The model under review builds one solid part; all positions refer to its coordinate system, in mm. A direction names the side the tool comes from. Coordinates: 2 decimals unless noted, no trailing zeros. Order: outer loops, then holes, each group sorted by start corner. A loop starts at its lowest first (then second) coordinate and runs counter-clockwise, first axis right, second up. Notation, with made-up numbers: M -40,41 L -4,41 A11 cw -4,53 Z; hole C 38.25,70.25 d1. An arc over 180 degrees is marked long. Write each question's results on one line, items separated by ' | '.
from build123d import *

# Parameters (mm, degrees)
SALIENTE_EXTRUIR1_DEPTH = 6.8
CROQUIS2_W              = 9
CROQUIS2_H              = 2.8
CORTAR_EXTRUIR1_DEPTH   = 18.969669092
REDONDEO1_R             = 0.5
REDONDEO2_R             = 0.5
REDONDEO3_R             = 0.5
REDONDEO4_R             = 0.5


with BuildPart() as part:
    # Croquis1 → Saliente-Extruir1 (new body)
    with BuildSketch(Plane(origin=(0, 0, 0), x_dir=(1, 0, 0), z_dir=(0, 1, 0))):
        with BuildLine():
            Line((0, 0), (0, 14))
            Line((0, 14), (1, 14))
            Line((1, 14), (1, 1.5))
            Line((1, 1.5), (3.5, 1.5))
            Line((3.5, 1.5), (3.5, 9.4))
            Line((3.5, 9.4), (1.5, 9.4))
            Line((1.5, 9.4), (1.5, 11.6))
            Line((1.5, 11.6), (3.5, 11.6))
            Line((3.5, 11.6), (3.5, 17.969669092))
            Line((3.5, 17.969669092), (4.5, 17.969669092))
            Line((4.5, 17.969669092), (4.5, 2.5))
            ThreePointArc((4.5, 2.5), (4.792893219, 1.792893219), (5.5, 1.5))
            Line((5.5, 1.5), (12.5, 1.5))
            ThreePointArc((12.5, 1.5), (13.207106781, 1.792893219), (13.5, 2.5))
            Line((13.5, 2.5), (13.5, 17.969669092))
            Line((13.5, 17.969669092), (14.5, 17.969669092))
            Line((14.5, 17.969669092), (14.5, 11.6))
            Line((14.5, 11.6), (16.5, 11.6))
            Line((16.5, 11.6), (16.5, 9.4))
            Line((16.5, 9.4), (14.5, 9.4))
            Line((14.5, 9.4), (14.5, 1.5))
            Line((14.5, 1.5), (17, 1.5))
            Line((17, 1.5), (17, 14))
            Line((17, 14), (18, 14))
            Line((18, 14), (18, 0))
            Line((18, 0), (0, 0))
        make_face()
    extrude(amount=SALIENTE_EXTRUIR1_DEPTH)

    # Croquis2 → Cortar-Extruir1 (cut, through all)
    with BuildSketch(Plane.XY):
        with Locations((9, 3.4)):
            Rectangle(CROQUIS2_W, CROQUIS2_H)
    extrude(amount=-CORTAR_EXTRUIR1_DEPTH, mode=Mode.SUBTRACT)

    # Redondeo1
    redondeo1_edges = [part.edges().sort_by_distance(p)[0] for p in [
        (16.5, 3.4, -11.6),
    ]]
    fillet(redondeo1_edges, radius=REDONDEO1_R)

    # Redondeo2
    redondeo2_edges = [part.edges().sort_by_distance(p)[0] for p in [
        (16.5, 3.4, -9.4),
    ]]
    fillet(redondeo2_edges, radius=REDONDEO2_R)

    # Redondeo3
    redondeo3_edges = [part.edges().sort_by_distance(p)[0] for p in [
        (1.5, 3.4, -9.4),
    ]]
    fillet(redondeo3_edges, radius=REDONDEO3_R)

    # Redondeo4
    redondeo4_edges = [part.edges().sort_by_distance(p)[0] for p in [
        (1.5, 3.4, -11.6),
    ]]
    fillet(redondeo4_edges, radius=REDONDEO4_R)


solid = part.part
1) Take a section at A-A on x = 9. State the section outline as (y, z) points.
Solutions:
outline: M 0,-1.5 L 2,-1.5 L 2,0 L 0,0 Z; M 4.8,-1.5 L 6.8,-1.5 L 6.8,0 L 4.8,0 Z
2) Take a section at C-C on z = -9. State the section outline as (x, y) points.
Solutions:
outline: M 0,0 L 1,0 L 1,6.8 L 0,6.8 Z; M 3.5,0 L 4.5,0 L 4.5,6.8 L 3.5,6.8 Z; M 13.5,0 L 14.5,0 L 14.5,6.8 L 13.5,6.8 Z; M 17,0 L 18,0 L 18,6.8 L 17,6.8 Z
3) For faces 4 (the flat face through (14, 3, -17.97)), 5 (the flat face through (14.5, 3, -15)), 6 (the flat face through (9, 5, 0)), 7 (the flat face through (3, 3, -9.4)), 8 (the flat face through (17.5, 3.4, -14)), list the 3-axis set-ups (+Z, -Z, +X, -X, +Y, -Y) from which the entire face can be reached by the end or side of a thin tool; tool diameter is ignored.
Solutions:
face 4: -Z, +X, -X, +Y, -Y | face 5: -Z, +Y, -Y | face 6: +Z, +X, -X, +Y, -Y | face 7: +Y, -Y | face 8: -Z, +X, +Y, -Y
4) To check wall thickness, follow line 1 along X through (y, z) = (4, -8); line 2 along Z through (x, y) = (2, 4.75); line 3 along X through (y, z) = (1.5, -10.75). State the ranges of each line that lie inside material, in increasing order.
Solutions:
line 1: 0 to 1, 3.5 to 4.5, 13.5 to 14.5, 17 to 18 | line 2: -11.6 to -9.4, -1.5 to 0 | line 3: 0 to 1, 1.5 to 4.5, 13.5 to 16.5, 17 to 18
5) The part is to be moulded in two halves that separate along Y. For faces 1 (the flat face through (14, 6.8, -7)), 2 (the flat face through (15, 3, -11.6)), 3 (the flat face through (9, 2, -1)), say which applies: pulls with the +Y half, pulls with the -Y half, needs draft (parallel to the pull), parting line crosses it, or undercut.
Solutions:
face 1: pulls with the +Y half | face 2: needs draft | face 3: undercut
6) Take a section at B-B on y = 4. State the section outline as (x, z) points, plus the area to 3 significant figures.
Solutions:
outline: M 0,-14 L 1,-14 L 1,-1.5 L 3.5,-1.5 L 3.5,-9.4 L 2,-9.4 A0.5 ccw 1.5,-9.9 L 1.5,-11.1 A0.5 ccw 2,-11.6 L 3.5,-11.6 L 3.5,-17.97 L 4.5,-17.97 L 4.5,0 L 0,0 Z; M 13.5,-17.97 L 14.5,-17.97 L 14.5,-11.6 L 16,-11.6 A0.5 ccw 16.5,-11.1 L 16.5,-9.9 A0.5 ccw 16,-9.4 L 14.5,-9.4 L 14.5,-1.5 L 17,-1.5 L 17,-14 L 18,-14 L 18,0 L 13.5,0 Z | area: 80.0 mm2
7) For pin 1 (4 mm diameter, centred on x = 10.5, y = 6, fed in from -Z); pin 2 (1.6 mm diameter, centred on x = 15.5, y = 4, fed in from -Z); pin 3 (1 mm diameter, centred on y = 5.5, z = -13, fed in from -X), all flat-tipped, find the tip position at first contact; note any pin that passes through.
Solutions:
pin 1: z = -1.5 | pin 2: z = -11.6 | pin 3: x = 0
8) Take a section at D-D on x = 3. State the section outline as (y, z) points, plus the area to 3 significant figures.
Solutions:
outline: M 0,-11.6 L 6.8,-11.6 L 6.8,-9.4 L 0,-9.4 Z; M 0,-1.5 L 6.8,-1.5 L 6.8,0 L 0,0 Z | area: 25.2 mm2
